Here's how the part is built. I have some questions about the finished solid (model axes, mm). Round coordinates to 2 decimals unless told otherwise and drop trailing zeros. Write each loop counter-clockwise with the first axis right and the second up, starting at its lowest first coordinate (ties: lowest second). Pieces come first, ordered by that corner, then holes. Notation, with made-up numbers: (54.25, -26.75) - (102.25, -26.75) arc R16 cw to (102.25, -5.75) - close; hole circle Ø4 at (-34.5, 19). An arc over 180 degrees is marked (long way). Write item = value, one per line. Start each with the question number.
Item 1: If we section it at A-A (x = -12.7): Please give me the cut outline in (y, z), and give its area (3 significant figures).
Item 2: If I drill on line 1 along Z through (x, y) = (-139.7, 14.25); line 2 along X through (y, z) = (11.5, 186); line 3 along Z through (x, y) = (-136, 5.25), over which ranges is the centre line in solid material (lowest first)? Write a range as [from, to].
Item 3: If we section it at B-B (z = 139.7): Please give me the cut outline in (x, y).
Item 4: If we section it at D-D (x = -139.7): Please give me the cut outline in (y, z).
Item 5: If we section it at C-C (z = 190.5): Please give me the cut outline in (x, y), and give its area (3 significant figures).
Autodesk Inventor part; units mm, degrees
ref_plane "YZ Plane" through (0, 0, 0) normal (1, 0, 0) x (0, 1, 0)
ref_plane "XZ Plane" through (0, 0, 0) normal (0, 1, 0) x (-1, 0, 0)
ref_plane "XY Plane" through (0, 0, 0) normal (0, 0, 1) x (1, 0, 0)
sketch "Sketch1" plane through (0, 0, 0) normal (0, 1, 0) x (-1, 0, 0)
  line L0 (0, 0) -> (152.4, 0)
  line L1 (152.4, 0) -> (152.4, 203.2)
  line L2 (152.4, 203.2) -> (0, 203.2)
  line L3 (0, 203.2) -> (0, 0)
  circle A0 centre (12.7, 190.5) radius 7.9375
  circle A1 centre (139.7, 190.5) radius 7.9375
  circle A2 centre (139.7, 12.7) radius 7.9375
  circle A3 centre (12.7, 12.7) radius 7.9375
  circle A4 centre (114.3, 190.5) radius 3.302
  circle A5 centre (38.1, 190.5) radius 3.302
  circle A6 centre (114.3, 12.7) radius 3.302
  circle A7 centre (38.1, 12.7) radius 3.302
  circle A8 centre (139.7, 139.7) radius 3.302
  circle A9 centre (139.7, 63.5) radius 3.302
  circle A10 centre (20.32, 168.148) radius 1.524
  circle A11 centre (20.32, 153.924) radius 1.524
  circle A12 centre (20.32, 128.524) radius 1.524
  circle A13 centre (20.32, 114.3) radius 1.524
  circle A14 centre (20.32, 88.9) radius 1.524
  circle A15 centre (20.32, 74.676) radius 1.524
  circle A16 centre (18.796, 49.276) radius 1.524
  circle A17 centre (18.796, 35.052) radius 1.524
  dimension "d0" = 152.4
  dimension "d1" = 203.2
  dimension "d40" = 15.875
  dimension "d41" = 15.875
  dimension "d42" = 15.875
  dimension "d43" = 15.875
  dimension "d44" = 12.7
  dimension "d45" = 12.7
  dimension "d46" = 12.7
  dimension "d47" = 12.7
  dimension "d48" = 12.7
  dimension "d49" = 12.7
  dimension "d50" = 12.7
  dimension "d51" = 12.7
  dimension "d52" = 177.8
  dimension "d53" = 127
  dimension "d54" = 6.604
  dimension "d55" = 6.604
  dimension "d56" = 25.4
  dimension "d57" = 25.4
  dimension "d58" = 12.7
  dimension "d59" = 12.7
  dimension "d60" = 6.604
  dimension "d61" = 6.604
  dimension "d62" = 12.7
  dimension "d63" = 12.7
  dimension "d64" = 25.4
  dimension "d65" = 25.4
  dimension "d66" = 6.604
  dimension "d67" = 6.604
  dimension "d68" = 50.8
  dimension "d69" = 50.8
  dimension "d70" = 12.7
  dimension "d71" = 12.7
  dimension "d72" = 3.048
  dimension "d73" = 3.048
  dimension "d74" = 3.048
  dimension "d75" = 3.048
  dimension "d76" = 3.048
  dimension "d77" = 3.048
  dimension "d78" = 20.32
  dimension "d79" = 20.32
  dimension "d80" = 20.32
  dimension "d81" = 20.32
  dimension "d82" = 20.32
  dimension "d83" = 20.32
  dimension "d84" = 22.352
  dimension "d85" = 14.224
  dimension "d86" = 25.4
  dimension "d87" = 14.224
  dimension "d88" = 25.4
  dimension "d89" = 14.224
  dimension "d90" = 3.048
  dimension "d91" = 3.048
  dimension "d92" = 25.4
  dimension "d93" = 14.224
extrude "Extrusion2" add sketch "Sketch1" along normal blind 25.4
properties part number "CasingBottomWithSlots"
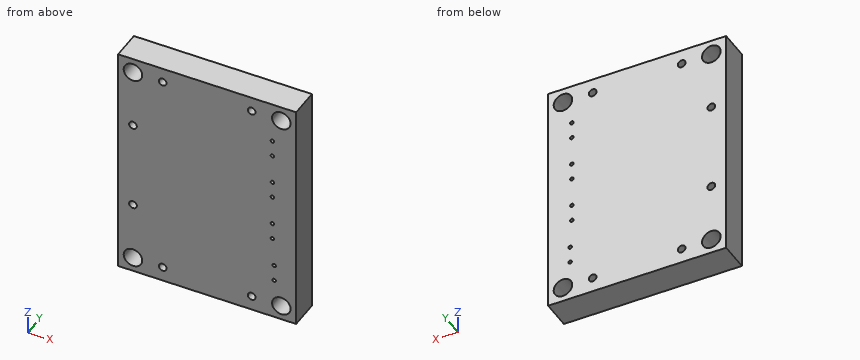
Reply:
q1.outline = (0, 0) - (25.4, 0) - (25.4, 4.76) - (0, 4.76) - close; (0, 20.64) - (25.4, 20.64) - (25.4, 182.56) - (0, 182.56) - close; (0, 198.44) - (25.4, 198.44) - (25.4, 203.2) - (0, 203.2) - close
q1.area = 4,350 mm2
q2.line_1 = [0, 4.76], [20.64, 60.2], [66.8, 136.4], [143, 182.56], [198.44, 203.2]
q2.line_2 = [-152.4, -146.24], [-133.16, -19.24], [-6.16, 0]
q2.line_3 = [0, 5.68], [19.72, 183.48], [197.52, 203.2]
q3.outline = (-152.4, 0) - (-143, 0) - (-143, 25.4) - (-152.4, 25.4) - close; (-136.4, 0) - (0, 0) - (0, 25.4) - (-136.4, 25.4) - close
q4.outline = (0, 0) - (25.4, 0) - (25.4, 4.76) - (0, 4.76) - close; (0, 20.64) - (25.4, 20.64) - (25.4, 60.2) - (0, 60.2) - close; (0, 66.8) - (25.4, 66.8) - (25.4, 136.4) - (0, 136.4) - close; (0, 143) - (25.4, 143) - (25.4, 182.56) - (0, 182.56) - close; (0, 198.44) - (25.4, 198.44) - (25.4, 203.2) - (0, 203.2) - close
q5.outline = (-152.4, 0) - (-147.64, 0) - (-147.64, 25.4) - (-152.4, 25.4) - close; (-131.76, 0) - (-117.6, 0) - (-117.6, 25.4) - (-131.76, 25.4) - close; (-111, 0) - (-41.4, 0) - (-41.4, 25.4) - (-111, 25.4) - close; (-34.8, 0) - (-20.64, 0) - (-20.64, 25.4) - (-34.8, 25.4) - close; (-4.76, 0) - (0, 0) - (0, 25.4) - (-4.76, 25.4) - close
q5.area = 2,730 mm2
